from build123d import *

# Parameters (mm, degrees)
F0_W     = 20
F0_H     = 20
F0_R     = 3
F1_DEPTH = 10
F3_DEPTH = 20
F4_R     = 1


with BuildPart() as f1:
    # F0 (on Top) → F1 (new body)
    with BuildSketch(Plane.XY):
        Rectangle(F0_W, F0_H)
        Circle(F0_R, mode=Mode.SUBTRACT)
    extrude(amount=F1_DEPTH)

    # F2 (on face) → F3 (cut, through all)
    with BuildSketch(Plane.YZ.offset(10)):
        Polygon((-7, 5), (-10, 8), (-10, 2), align=None)
    extrude(amount=-F3_DEPTH, mode=Mode.SUBTRACT)

    # F4
    f4_edges = [f1.edges().sort_by_distance(p)[0] for p in [
        (0, -7, 5),
        (0, -10, 8),
        (0, -10, 2),
    ]]
    fillet(f4_edges, radius=F4_R)


solid = f1.part
The listing builds one solid part. Answer for the finished solid, in the listing's coordinates (mm). A direction names the side the tool comes from. Give positions to 0.01 mm unless a question says otherwise; leave off trailing zeros. Write each loop counter-clockwise with the first axis right and the second up, starting at its lowest first coordinate (ties: lowest second). Pieces come first, ordered by that corner, then holes. Notation, with made-up numbers: (-28, 5.25) - (-18, 5.25) arc R18 ccw to (-18, 40.25) - close; hole circle Ø10 at (28, -16). An arc over 180 degrees is marked (long way). One line per question, with ' | ' between items. Start each with the question number.
1. Section C-C, the plane y = 0.5 is taken. Determine the outline of the cut face in (x, z).
2. Straight lines are drawn through the part: line 1 (Y direction, x = 0, z = 5.25); line 2 (Y direction, x = 0, z = 4.5); line 3 (X direction, y = 1.5, z = 6.25). For each, find the intervals that lie inside material, in ascending order.
3. Section A-A, the plane x = 0 is taken. Determine the outline of the cut face in (y, z).
4. Section B-B, the plane z = 4 is taken. Determine the outline of the cut face in (x, y), then the cut area to 3 significant figures.
5. Determine the mould class of faces 1 (the face through (-3, 0, 5)), 2 (the face through (10, 0, 5)), 3 (the face through (-0.14, -7.414, 5.011)) for opening direction X: +X half, -X half, draft (parallel to the pull), parting line (faces both ways), or undercut.
6. Section D-D, the plane x = -4.75 is taken. Determine the outline of the cut face in (y, z), then the cut area to 3 significant figures.
7. Given P1, Ø4, axis at x = 5, z = 5.5, coming from the -Y side, flat-ended and moving along its own axis, determine where the tip first touches the part or whether it passes through.
8. For faces 4 (the face through (0, 10, 5)), 5 (the face through (0, -9, 7)), determine the directions among +Z, -Z, +X, -X, +Y, -Y from which every point of the face is accessible in a straight line to the end or side of a thin tool.
Result:
1) outline: (-10, 0) - (-2.96, 0) - (-2.96, 10) - (-10, 10) - close; (2.96, 0) - (10, 0) - (10, 10) - (2.96, 10) - close
2) line 1: y = -7.45 to -3, 3 to 10 | line 2: y = -7.55 to -3, 3 to 10 | line 3: x = -10 to -2.6, 2.6 to 10
3) outline: (-10, 0) - (-3, 0) - (-3, 10) - (-10, 10) - (-10, 8.41) arc R1 ccw to (-9.71, 7.71) - (-7.71, 5.71) arc R1 cw to (-7.71, 4.29) - (-9.71, 2.29) arc R1 ccw to (-10, 1.59) - close; (3, 0) - (10, 0) - (10, 10) - (3, 10) - close
4) outline: (-10, -8) - (10, -8) - (10, 10) - (-10, 10) - close; hole circle Ø6 at (0, 0) | area: 332 mm2
5) face 1: undercut | face 2: +X half | face 3: draft
6) outline: (-10, 0) - (10, 0) - (10, 10) - (-10, 10) - (-10, 8.41) arc R1 ccw to (-9.71, 7.71) - (-7.71, 5.71) arc R1 cw to (-7.71, 4.29) - (-9.71, 2.29) arc R1 ccw to (-10, 1.59) - close | area: 191 mm2
7) P1: stops at y = -9.5
8) face 4: +Z, -Z, +X, -X, +Y | face 5: +X, -X, -Y
